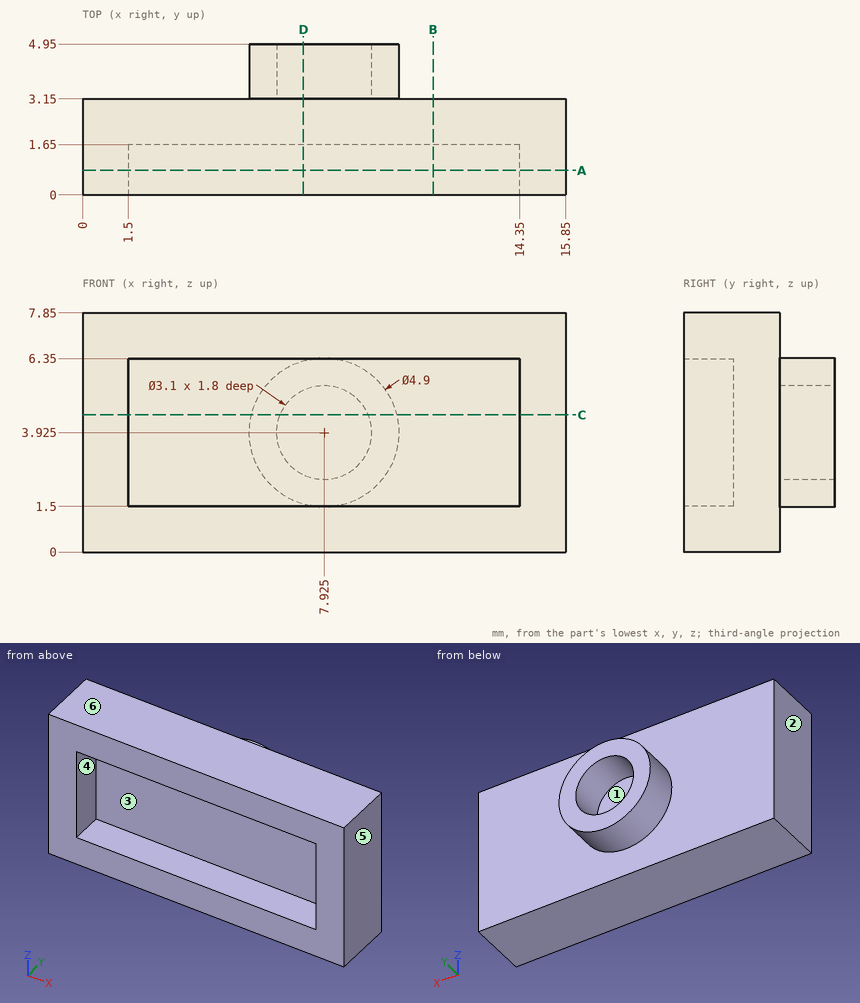
Answer from the drawing. Dimensions are ordinates in mm from the lowest x, y and z of the part. A direction names the side the tool comes from. Round coordinates to 2 decimals unless told otherwise and drop trailing zeros. Write each loop counter-clockwise with the first axis right and the second up, starting at its lowest first coordinate (ties: lowest second). Pieces come first, ordered by that corner, then holes. Notation, with made-up numbers: (10, 48) -> (29, 48) arc R36 ccw to (29, 87) -> close; hole circle Ø5 at (-33, 35). An arc over 180 degrees is marked (long way). Write each question's results on one line, items separated by ' | '.
1) Consider line 1 along X through (y, z) = (1.25, 4.25); line 2 along Z through (x, y) = (3.25, 1.2); line 3 along X through (y, z) = (3.9, 4). Determine where each line is inside the solid, lowest interval first. Write a range as [from, to].
Findings:
line 1: x = [0, 1.5], [14.35, 15.85] | line 2: z = [0, 1.5], [6.35, 7.85] | line 3: x = [5.48, 6.38], [9.47, 10.37]
2) The part is cut by section C-C (z = 4.5). Write down the section's boundary in (x, y), and give its area (3 significant figures).
Findings:
outline: (0, 0) -> (1.5, 0) -> (1.5, 1.65) -> (14.35, 1.65) -> (14.35, 0) -> (15.85, 0) -> (15.85, 3.15) -> (10.31, 3.15) -> (10.31, 4.95) -> (9.36, 4.95) -> (9.36, 3.15) -> (6.49, 3.15) -> (6.49, 4.95) -> (5.54, 4.95) -> (5.54, 3.15) -> (0, 3.15) -> close | area: 32.1 mm²
3) For a pull along X with two mould halves and no side action, classify the marked faces 4, 5 and 6 as +X half, -X half, draft (parallel to the pull), parting line (faces both ways), or undercut.
Findings:
face 4: undercut | face 5: +X half | face 6: draft
4) The part is cut by section B-B (x = 11.5). Write down the section's boundary in (y, z).
Findings:
outline: (0, 0) -> (3.15, 0) -> (3.15, 7.85) -> (0, 7.85) -> (0, 6.35) -> (1.65, 6.35) -> (1.65, 1.5) -> (0, 1.5) -> close
5) The part is cut by section D-D (x = 7.25). Write down the section's boundary in (y, z).
Findings:
outline: (0, 0) -> (3.15, 0) -> (3.15, 1.57) -> (4.95, 1.57) -> (4.95, 2.53) -> (3.15, 2.53) -> (3.15, 5.32) -> (4.95, 5.32) -> (4.95, 6.28) -> (3.15, 6.28) -> (3.15, 7.85) -> (0, 7.85) -> (0, 6.35) -> (1.65, 6.35) -> (1.65, 1.5) -> (0, 1.5) -> close
6) Flat-ended cylindrical pins translate along their axes: pin 1 (1.9 mm diameter, centred on x = 7.925, z = 3.925, fed in from -Y); pin 2 (1.5 mm diameter, centred on x = 5.5, z = 1, fed in from +Y). Find the tip coordinate at first contact, or state that the pin passes through.
Findings:
pin 1: stops at y = 1.65 | pin 2: stops at y = 3.15
7) The part is cut by section A-A (y = 0.8). Write down the section's boundary in (x, z), and give its area (3 significant figures).
Findings:
outline: (0, 0) -> (15.85, 0) -> (15.85, 7.85) -> (0, 7.85) -> close; hole (1.5, 1.5) -> (14.35, 1.5) -> (14.35, 6.35) -> (1.5, 6.35) -> close | area: 62.1 mm²
8) Which of the six approach directions +Z, -Z, +X, -X, +Y, -Y give full straight-line access (tool end or side, diameter ignored) to the marked faces 1, 2 and 3?
Findings:
face 1: +Y | face 2: +Z, -Z, -X, +Y, -Y | face 3: -Y
